```python
from build123d import *

# Parameters (mm, degrees)
BASE_EXTRUDE_DEPTH = 12.7


with BuildPart() as part:
    # Sketch1 → Base-Extrude (new, symmetric)
    with BuildSketch(Plane.XY):
        with BuildLine():
            Line((-20.6375, 21.1074), (-20.6375, 11.73965134))
            ThreePointArc((-20.6375, 11.73965134), (-19.1389, 9.144), (-20.6375, 6.54834866))
            Line((-20.6375, 6.54834866), (-20.6375, -6.54834866))
            ThreePointArc((-20.6375, -6.54834866), (-19.1389, -9.144), (-20.6375, -11.73965134))
            Line((-20.6375, -11.73965134), (-20.6375, -17.1704))
            ThreePointArc((-20.6375, -17.1704), (-20.198570222, -18.230070222), (-19.1389, -18.669))
            Line((-19.1389, -18.669), (19.1389, -18.669))
            ThreePointArc((19.1389, -18.669), (20.198570222, -18.230070222), (20.6375, -17.1704))
            Line((20.6375, -17.1704), (20.6375, -11.73965134))
            ThreePointArc((20.6375, -11.73965134), (19.1389, -9.144), (20.6375, -6.54834866))
            Line((20.6375, -6.54834866), (20.6375, 6.54834866))
            ThreePointArc((20.6375, 6.54834866), (19.1389, 9.144), (20.6375, 11.73965134))
            Line((20.6375, 11.73965134), (20.6375, 21.1074))
            ThreePointArc((20.6375, 21.1074), (20.198570222, 22.167070222), (19.1389, 22.606))
            Line((19.1389, 22.606), (12.6111, 22.606))
            ThreePointArc((12.6111, 22.606), (11.551429778, 22.167070222), (11.1125, 21.1074))
            Line((11.1125, 21.1074), (11.1125, 16.256))
            Line((11.1125, 16.256), (12.6111, 16.256))
            Line((12.6111, 16.256), (12.6111, 21.1074))
            Line((12.6111, 21.1074), (19.1389, 21.1074))
            Line((19.1389, 21.1074), (19.1389, 12.494971471))
            ThreePointArc((19.1389, 12.494971471), (17.6403, 9.144), (19.1389, 5.793028529))
            Line((19.1389, 5.793028529), (19.1389, -5.793028529))
            ThreePointArc((19.1389, -5.793028529), (17.6403, -9.144), (19.1389, -12.494971471))
            Line((19.1389, -12.494971471), (19.1389, -17.1704))
            Line((19.1389, -17.1704), (-19.1389, -17.1704))
            Line((-19.1389, -17.1704), (-19.1389, -12.494971471))
            ThreePointArc((-19.1389, -12.494971471), (-17.6403, -9.144), (-19.1389, -5.793028529))
            Line((-19.1389, -5.793028529), (-19.1389, 5.793028529))
            ThreePointArc((-19.1389, 5.793028529), (-17.6403, 9.144), (-19.1389, 12.494971471))
            Line((-19.1389, 12.494971471), (-19.1389, 21.1074))
            Line((-19.1389, 21.1074), (-12.6111, 21.1074))
            Line((-12.6111, 21.1074), (-12.6111, 16.256))
            Line((-12.6111, 16.256), (-11.1125, 16.256))
            Line((-11.1125, 16.256), (-11.1125, 21.1074))
            ThreePointArc((-11.1125, 21.1074), (-11.551429778, 22.167070222), (-12.6111, 22.606))
            Line((-12.6111, 22.606), (-19.1389, 22.606))
            ThreePointArc((-19.1389, 22.606), (-20.198570222, 22.167070222), (-20.6375, 21.1074))
        make_face()
    extrude(amount=BASE_EXTRUDE_DEPTH, both=True)


solid = part.part
```
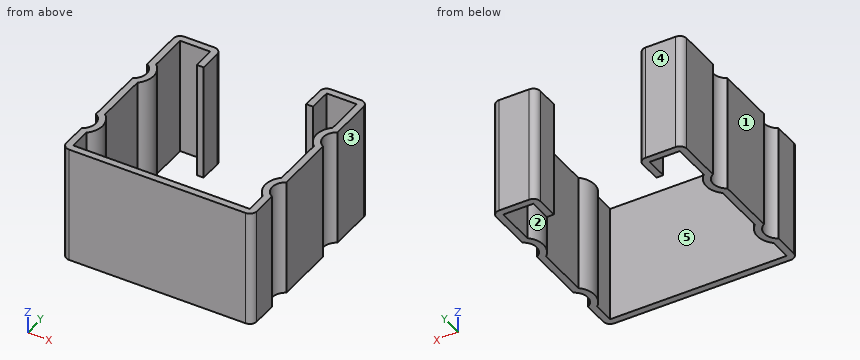
Verification items for the finished model (mm, model axes). Face numbers are marked on the shaded views. A direction names the side the tool comes from. Round coordinates to 2 decimals unless told otherwise and drop trailing zeros. Write each loop counter-clockwise with the first axis right and the second up, starting at its lowest first coordinate (ties: lowest second). Pieces come first, ordered by that corner, then holes.
1. Draft check along X on the marked faces 3, 4 and 5. Enter one of: +X half, -X half, draft (parallel to the pull), parting line (faces both ways), or undercut.
2. Section check C-C on x = 2. Enter the section's corners in (y, z).
3. Gauge pin test, flat end, axial feed: P1, Ø2, axis at x = 5, z = 2, coming from the +Y side. Record the tip position at first contact, or that the pin passes through.
4. Section check B-B on y = -4.5. Enter the section's corners in (x, z), plus the area to 3 significant figures.
5. Scan lines: L1, parallel to X at y = 20.5, z = 8; L2, parallel to Y at x = 16, z = -11; L3, parallel to X at y = 14, z = -2.25. Record each from-to range of solid material in increasing order.
6. Access from +Z, -Z, +X, -X, +Y, -Y to the whole of each face (thin tool, end or side, straight path). Record for the marked faces 1 and 2.
7. Section check A-A on x = -13.5. Enter the section's corners in (y, z), plus the area to 3 significant figures.
Answer:
1. face 3: +X half
1. face 4: draft
1. face 5: undercut
2. outline: (-18.67, -12.7) - (-17.17, -12.7) - (-17.17, 12.7) - (-18.67, 12.7) - close
3. P1: stops at y = -17.17
4. outline: (-20.64, -12.7) - (-19.14, -12.7) - (-19.14, 12.7) - (-20.64, 12.7) - close; (19.14, -12.7) - (20.64, -12.7) - (20.64, 12.7) - (19.14, 12.7) - close
4. area: 76.1 mm2
5. L1: x = -20.64 to -19.14, -12.61 to -11.11, 11.11 to 12.61, 19.14 to 20.64
5. L2: y = -18.67 to -17.17, 21.11 to 22.61
5. L3: x = -20.64 to -19.14, 19.14 to 20.64
6. face 1: +Z, -Z, -X, +Y, -Y
6. face 2: +Z, -Z
7. outline: (-18.67, -12.7) - (-17.17, -12.7) - (-17.17, 12.7) - (-18.67, 12.7) - close; (21.11, -12.7) - (22.61, -12.7) - (22.61, 12.7) - (21.11, 12.7) - close
7. area: 76.1 mm2
